from build123d import *

# Parameters (mm, degrees)
SKETCH1_W           = 8
SKETCH1_H           = 11
SKETCH1_R           = 2.555
BOSS_EXTRUDE1_DEPTH = 1.35
SKETCH2_W           = 0.77
SKETCH2_H           = 0.5
BOSS_EXTRUDE2_DEPTH = 15
BOSS_EXTRUDE3_DEPTH = 2.7


with BuildPart() as part:
    # Sketch1 → Boss-Extrude1 (new, symmetric)
    with BuildSketch(Plane.XY):
        Rectangle(SKETCH1_W, SKETCH1_H)
        with Locations(Location((0, -1.7, 0), (0, 0, 180))):
            Circle(SKETCH1_R, mode=Mode.SUBTRACT)
    extrude(amount=BOSS_EXTRUDE1_DEPTH, both=True)

    # Sketch2 → Boss-Extrude2 (add)
    with BuildSketch(Plane(origin=(0, 5.5, 0), x_dir=(1, 0, 0), z_dir=(0, 1, 0))):
        Rectangle(SKETCH2_W, SKETCH2_H)
        with Locations((-2, 0)):
            Rectangle(SKETCH2_W, SKETCH2_H)
        with Locations((2, 0)):
            Rectangle(SKETCH2_W, SKETCH2_H)
    extrude(amount=BOSS_EXTRUDE2_DEPTH)

    # Sketch4 → Boss-Extrude3 (add)
    with BuildSketch(Plane.XY.offset(1.35)):
        with BuildLine():
            Line((-0.6, 0.823242633), (-0.6, -0.056071778))
            ThreePointArc((-0.6, -0.056071778), (-1.515544457, -0.825), (-1.723683602, -2.002348869))
            Line((-1.723683602, -2.002348869), (-2.48519222, -2.442006074))
            ThreePointArc((-2.48519222, -2.442006074), (-2.246122223, -0.40320073), (-0.6, 0.823242633))
        make_face()
        with BuildLine():
            Line((0.6, 0.823242633), (0.6, -0.056071778))
            ThreePointArc((0.6, -0.056071778), (1.515544457, -0.825), (1.723683602, -2.002348869))
            Line((1.723683602, -2.002348869), (2.48519222, -2.442006074))
            ThreePointArc((2.48519222, -2.442006074), (2.246122223, -0.40320073), (0.6, 0.823242633))
        make_face()
        with BuildLine():
            Line((1.88519222, -3.481236559), (1.123683602, -3.041579353))
            ThreePointArc((1.123683602, -3.041579353), (0, -3.45), (-1.123683602, -3.041579353))
            Line((-1.123683602, -3.041579353), (-1.88519222, -3.481236559))
            ThreePointArc((-1.88519222, -3.481236559), (0, -4.29359854), (1.88519222, -3.481236559))
        make_face()
    extrude(amount=-BOSS_EXTRUDE3_DEPTH)


solid = part.part
CAD build for the part. Positions are in the model's coordinates, mm. A direction names the side the tool comes from. Give positions to 0.01 mm unless a question says otherwise; leave off trailing zeros. Order: outer loops, then holes, each group sorted by start corner. A loop starts at its lowest first (then second) coordinate and runs counter-clockwise, first axis right, second up. Notation, with made-up numbers: (14, 29.5) - (48, 29.5) arc R26 cw to (48, 64.5) - close; hole circle Ø10 at (19.25, -28). An arc over 180 degrees is marked (long way). Write each question's results on one line, items separated by ' | '.
1. Saw through at B-B on z = -0.8. List the corners of the cut face in (x, y) (3 decimals).
Calculated:
outline: (-4, -5.5) - (4, -5.5) - (4, 5.5) - (-4, 5.5) - close; hole (-2.451, -2.422) arc R2.555 ccw to (-1.851, -3.461) - (-1.124, -3.042) arc R1.75 ccw to (1.124, -3.042) - (1.851, -3.461) arc R2.555 ccw to (2.451, -2.422) - (1.724, -2.002) arc R1.75 ccw to (0.6, -0.056) - (0.6, 0.784) arc R2.555 ccw to (-0.6, 0.784) - (-0.6, -0.056) arc R1.75 ccw to (-1.724, -2.002) - close
2. Probe L1, parallel to X at y = 9.5, z = -0.1 (3 decimals); L2, parallel to Y at x = 0, z = 0.3 (3 decimals); L3, parallel to Z at x = -2, y = 19. List the from-to ranges inside material, lowest first. Write a range as from..to.
Calculated:
L1: x = -2.385..-1.615, -0.385..0.385, 1.615..2.385 | L2: y = -5.5..-3.45, 0.855..5.5 | L3: z = -0.25..0.25
3. Pull direction Y, two halves, no side cores. Call faces 1 (the face through (0, -5.5, 0)), 2 (the face through (-4, 0, 0)), 3 (the face through (2.2, -3, 0)): released by +Y, released by -Y, zero draft, split by the parting line, or undercut.
Calculated:
face 1: released by -Y | face 2: zero draft | face 3: undercut
4. Saw through at A-A on y = 12.25. List the corners of the cut face in (x, z) (3 decimals), and give its area (4 significant figures).
Calculated:
outline: (-2.385, -0.25) - (-1.615, -0.25) - (-1.615, 0.25) - (-2.385, 0.25) - close; (-0.385, -0.25) - (0.385, -0.25) - (0.385, 0.25) - (-0.385, 0.25) - close; (1.615, -0.25) - (2.385, -0.25) - (2.385, 0.25) - (1.615, 0.25) - close | area: 1.155 mm2
5. Saw through at C-C on x = -3. List the corners of the cut face in (y, z), and give its area (3 significant figures).
Calculated:
outline: (-5.5, -1.35) - (5.5, -1.35) - (5.5, 1.35) - (-5.5, 1.35) - close | area: 29.7 mm2
6. Pin check, flat tips, straight feed: pin 1 (0.6 mm diameter, centred on y = 10, z = 0, fed in from +X) (3 decimals); pin 2 (1 mm diameter, centred on x = 0.5, z = -1, fed in from +Y); pin 3 (0.6 mm diameter, centred on y = 12.5, z = 0, fed in from -X) (3 decimals). Stop position of each tip, or through.
Calculated:
pin 1: stops at x = 2.385 | pin 2: stops at y = 5.5 | pin 3: stops at x = -2.385
7. 3-axis set-ups, long thin cutter, end or side, ignore diameter. For faces 4 (the face through (-1.5, -0.8, 0)), 5 (the face through (1, 0, 1.35)): which of +Z, -Z, +X, -X, +Y, -Y reach the whole face in a straight line?
Calculated:
face 4: +Z, -Z | face 5: +Z, +X, -X, +Y, -Y
